Build history of the part. All positions in model axes, mm. A direction names the side the tool comes from. Round coordinates to 2 decimals unless told otherwise and drop trailing zeros. Loops run counter-clockwise (first coordinate to the right, second up) from the corner with the lowest first, then second, coordinate; pieces in that order, holes last. Notation, with made-up numbers: (49, 7.5) -> (77, 7.5) arc R24 cw to (77, 21.5) -> close; hole circle Ø8 at (49, 39). An arc over 180 degrees is marked (long way). Put each result on its own line as item: value. Start each with the question number.
Item 1: Drill centre lines: probe 1 along Z at (x, y) = (5.5, 24); probe 2 along Z at (x, y) = (-4, 4.5); probe 3 along X at (y, z) = (3.5, 4.5). Where is each one in solid material? Low to high. Write a range as [from, to].
Item 2: Tool access for faces 1 (the flat face through (7, 28.448, 0)), 2 (the flat face through (7, 7.874, 0)), 3 (the flat face through (-3, 28.448, -6)), 4 (the flat face through (-3, 7.874, 6)): list every direction of +Z, -Z, +X, -X, +Y, -Y with a clear straight run to the whole face (end or side of a thin tool).
Item 3: Flat gauge pins, fed straight in: pin 1 Ø8 at (x, y) = (-5, 33.5) entering from -Z; pin 2 Ø0.9 at (x, z) = (7, 0.5) entering from +Y; pin 3 Ø5 at (x, y) = (4, 34.5) entering from -Z. Where does each tip first touch, or does it go through?
Item 4: Pull direction Y, two halves, no side cores. Call faces 5 (the cylindrical face through (-0.093, 3.882, -6.344)), 6 (the flat face through (-3, 28.448, 6)), 7 (the flat face through (3, 7.874, -6)): +Y half, -Y half, draft (parallel to the pull), parting line (faces both ways), or undercut.
Item 5: Cut at B-B, the plane z = 2.25. List the corners of the cut face in (x, y), plus the area to 3 significant figures.
Item 6: Cut at D-D, the plane y = 18. List the corners of the cut face in (x, z), plus the area to 3 significant figures.
Item 7: Cut at C-C, the plane x = -5. List the corners of the cut face in (y, z), plus the area to 3 significant figures.
Autodesk Inventor part; units mm, degrees
ref_plane "YZ Plane" through (0, 0, 0) normal (1, 0, 0) x (0, 1, 0)
ref_plane "XZ Plane" through (0, 0, 0) normal (0, 1, 0) x (-1, 0, 0)
ref_plane "XY Plane" through (0, 0, 0) normal (0, 0, 1) x (1, 0, 0)
sketch "Sketch1" plane through (0, 0, 0) normal (0, 1, 0) x (-1, 0, 0)
  line L0 (-3.6631, -6.3447) -> (-7.3262, 0)
  line L1 (-7.3262, 0) -> (-3.6631, 6.3447)
  line L2 (-3.6631, 6.3447) -> (3.6631, 6.3447)
  line L3 (3.6631, 6.3447) -> (7.3262, 0)
  line L4 (7.3262, 0) -> (3.6631, -6.3447)
  line L5 (3.6631, -6.3447) -> (-3.6631, -6.3447)
  point P0 (0, 0)
  point P1 (0, 0)
extrude "Extrusion1" add sketch "Sketch1" along normal blind 38.862
sketch "Sketch2" plane through (0, 38.862, 0) normal (0, 1, 0) x (1, 0, 0)
  circle A0 centre (0, 0) radius 6.3447
  line L0 (-3.6631, 6.3447) -> (-7.3262, 0)
  line L1 (-12.7498, -15.4851) -> (22.5218, -15.4851)
  line L2 (22.5218, -15.4851) -> (22.5218, 21.9986)
  line L3 (22.5218, 21.9986) -> (-12.7498, 21.9986)
  line L4 (-12.7498, 21.9986) -> (-12.7498, -15.4851)
extrude "Extrusion2" cut sketch "Sketch2" against normal blind 10.414
sketch "Sketch3" plane through (0, 0, 0) normal (0, -1, 0) x (1, 0, 0)
  circle A0 centre (0, 0) radius 6.3447
  line L0 (13.1193, 9.9547) -> (-18.5882, 9.9547)
  line L1 (-18.5882, 9.9547) -> (-18.5882, -22.736)
  line L2 (-18.5882, -22.736) -> (13.1193, -22.736)
  line L3 (13.1193, -22.736) -> (13.1193, 9.9547)
extrude "Extrusion3" cut sketch "Sketch3" against normal blind 7.874
properties part number "Elevator Gearbox Hex"
Reply:
1. probe 1: z = [-3.16, 3.16]
1. probe 2: z = [-4.92, 4.92]
1. probe 3: x = [-4.47, 4.47]
2. face 1: +X, +Y
2. face 2: +X, -Y
2. face 3: -Z, -X, +Y
2. face 4: +Z, -X, -Y
3. pin 1: stops at z = -6.27
3. pin 2: stops at y = 28.45
3. pin 3: stops at z = -6.16
4. face 5: draft
4. face 6: +Y half
4. face 7: -Y half
5. outline: (-6.03, 7.87) -> (-5.93, 7.87) -> (-5.93, 0) -> (5.93, 0) -> (5.93, 7.87) -> (6.03, 7.87) -> (6.03, 28.45) -> (5.93, 28.45) -> (5.93, 38.86) -> (-5.93, 38.86) -> (-5.93, 28.45) -> (-6.03, 28.45) -> close
5. area: 465 mm^2
6. outline: (-7.33, 0) -> (-3.66, -6.34) -> (3.66, -6.34) -> (7.33, 0) -> (3.66, 6.34) -> (-3.66, 6.34) -> close
6. area: 139 mm^2
7. outline: (0, -3.91) -> (7.87, -3.91) -> (7.87, -4.03) -> (28.45, -4.03) -> (28.45, -3.91) -> (38.86, -3.91) -> (38.86, 3.91) -> (28.45, 3.91) -> (28.45, 4.03) -> (7.87, 4.03) -> (7.87, 3.91) -> (0, 3.91) -> close
7. area: 309 mm^2
